Part model, mm, in its own coordinate system. A direction names the side the tool comes from. Coordinates: 2 decimals unless noted, no trailing zeros. Order: outer loops, then holes, each group sorted by start corner. A loop starts at its lowest first (then second) coordinate and runs counter-clockwise, first axis right, second up.
1) Cut at A-A (x = 0). List the corners of the cut face in (y, z), and give its area (3 significant figures).
2) Pin check, flat tips, straight feed: pin 1 Ø4 at (x, z) = (1, 2.5) entering from +Y; pin 2 Ø1.5 at (x, y) = (2.5, 77) entering from +Z. Stop position of each tip, or through.
3) Wall check: L1, parallel to X at y = 69, z = -0.5; L2, parallel to Z at x = 0.25, y = 16; L3, parallel to Y at x = 3.75, z = -1.25. Give the ranges that are in metal, low to high.
4) Cut at D-D (y = 4). List the corners of the cut face in (x, z).
5) Cut at B-B (z = 0). List the corners of the cut face in (x, y).
6) Tool access for faces 1 (the flat face through (1, -20, 2)), 2 (the flat face through (-1, 126.8, 2)), 3 (the flat face through (0, 146.8, 0)): list every direction of +Z, -Z, +X, -X, +Y, -Y with a clear straight run to the whole face (end or side of a thin tool).
7) Cut at C-C (y = 123.5). List the corners of the cut face in (x, z).
```python
from build123d import *

# Parameters (mm, degrees)
SKETCH_1_R      = 4
EXTRUDE_1_DEPTH = 106.8
SKETCH_2_R      = 3
EXTRUDE_2_DEPTH = 20
SKETCH_3_R      = 2
EXTRUDE_3_DEPTH = 20
EXTRUDE_START   = 20
SKETCH_4_R      = 3
EXTRUDE_4_DEPTH = 20
SKETCH_5_R      = 2
EXTRUDE_5_DEPTH = 20


with BuildPart() as part:
    # 草图1 → 凸台-拉伸1 (new body)
    with BuildSketch(Plane(origin=(0, 0, 0), x_dir=(1, 0, 0), z_dir=(0, 1, 0))):
        with Locations(Location((0, 0, 0), (0, 0, 270))):
            Circle(SKETCH_1_R)
    extrude(amount=EXTRUDE_1_DEPTH)

    # 草图2 → 凸台-拉伸2 (add)
    with BuildSketch(Plane(origin=(0, 106.8, 0), x_dir=(1, 0, 0), z_dir=(0, 1, 0))):
        with Locations(Location((0, 0, 0), (0, 0, 270))):
            Circle(SKETCH_2_R)
    extrude(amount=EXTRUDE_2_DEPTH)

    # 草图3 → 凸台-拉伸3 (add)
    with BuildSketch(Plane(origin=(0, 126.8, 0), x_dir=(1, 0, 0), z_dir=(0, 1, 0))):
        with Locations(Location((0, 0, 0), (0, 0, 270))):
            Circle(SKETCH_3_R)
    extrude(amount=EXTRUDE_3_DEPTH)

    # 草图4 → 凸台-拉伸4 (add)
    with BuildSketch(Plane.XZ.offset(EXTRUDE_START)):
        with Locations(Location((0, 0, 0), (0, 0, 90))):
            Circle(SKETCH_4_R)
    extrude(amount=-EXTRUDE_4_DEPTH)

    # 草图5 → 凸台-拉伸5 (add)
    with BuildSketch(Plane.XZ.offset(20).offset(EXTRUDE_START)):
        with Locations(Location((0, 0, 0), (0, 0, 90))):
            Circle(SKETCH_5_R)
    extrude(amount=-EXTRUDE_5_DEPTH)


solid = part.part
```
Geometry check:
1. outline: (-40, -2) - (-20, -2) - (-20, -3) - (0, -3) - (0, -4) - (106.8, -4) - (106.8, -3) - (126.8, -3) - (126.8, -2) - (146.8, -2) - (146.8, 2) - (126.8, 2) - (126.8, 3) - (106.8, 3) - (106.8, 4) - (0, 4) - (0, 3) - (-20, 3) - (-20, 2) - (-40, 2) - close
1. area: 1,250 mm2
2. pin 1: stops at y = 146.8
2. pin 2: stops at z = 3.6
3. L1: x = -3.97 to 3.97
3. L2: z = -3.99 to 3.99
3. L3: y = 0 to 106.8
4. outline: circle Ø8 at (0, 0)
5. outline: (-4, 0) - (-3, 0) - (-3, -20) - (-2, -20) - (-2, -40) - (2, -40) - (2, -20) - (3, -20) - (3, 0) - (4, 0) - (4, 106.8) - (3, 106.8) - (3, 126.8) - (2, 126.8) - (2, 146.8) - (-2, 146.8) - (-2, 126.8) - (-3, 126.8) - (-3, 106.8) - (-4, 106.8) - close
6. face 1: -Y
6. face 2: +Y
6. face 3: +Z, -Z, +X, -X, +Y
7. outline: circle Ø6 at (0, 0)
